from build123d import *

# Parameters (mm, degrees)
BOSS_EXTRUDE1_DEPTH      = 2
BOSS_EXTRUDE1_DEPTH_BACK = 5
SKETCH3_R                = 4
BOSS_EXTRUDE2_DEPTH      = 5
BOSS_EXTRUDE2_DEPTH_BACK = 2
SKETCH2_R                = 4
BOSS_EXTRUDE3_START      = -13.929206
SKETCH4_R                = 3.5
BOSS_EXTRUDE3_DEPTH      = 27.858412
CUT_EXTRUDE1_DEPTH       = 29.057975838
CUT_EXTRUDE1_DEPTH_BACK  = 5
SKETCH5_R                = 3
CUT_EXTRUDE2_DEPTH       = 29.057975747
CUT_EXTRUDE2_DEPTH_BACK  = 5
SKETCH6_R                = 3
SKETCH7_R                = 1.6
CUT_EXTRUDE3_DEPTH       = 33.668792587
SKETCH8_R                = 1.6
CUT_EXTRUDE4_DEPTH       = 33.668792494
SPLIT1_START             = -4.0000001
SPLIT1_OUTLINE_W         = 20
SPLIT1_OUTLINE_H         = 8.75
SPLIT1_DEPTH             = 0.5000001
SPLIT1_START_2           = 3.5
SPLIT1_2_OUTLINE_W       = 20
SPLIT1_2_OUTLINE_H       = 8.75
SPLIT1_2_DEPTH           = 0.5
SPLIT1_START_3           = -16.25
SPLIT1_3_DEPTH           = 7
SPLIT1_START_4           = 9.25
SPLIT1_4_DEPTH           = 7
SPLIT1_5_DEPTH           = 7
SPLIT1_6_DEPTH           = 7


# Read off the part's stored shape, not the designer's step: Split1
with BuildPart() as part:
    # Sketch3 → Boss-Extrude1 (new, two sides: drawn at the far end of the back side and taken through both)
    with BuildSketch(Plane(origin=(-7, 0, 14.25), x_dir=(1, 0, 0), z_dir=(0, 0, 1)).offset(-BOSS_EXTRUDE1_DEPTH_BACK)):
        Circle(SKETCH3_R)
    extrude(amount=BOSS_EXTRUDE1_DEPTH + BOSS_EXTRUDE1_DEPTH_BACK)



with BuildPart() as body_2:
    # Sketch2 → Boss-Extrude2 (new, two sides: drawn at the far end of the back side and taken through both)
    with BuildSketch(Plane(origin=(7, 0, -14.25), x_dir=(1, 0, 0), z_dir=(0, 0, 1)).offset(-BOSS_EXTRUDE2_DEPTH_BACK)):
        Circle(SKETCH2_R)
    extrude(amount=BOSS_EXTRUDE2_DEPTH + BOSS_EXTRUDE2_DEPTH_BACK)


with BuildPart() as part_1:
    add(part.part)

    add(body_2.part)  # Boss-Extrude3 merges body 2
    # Sketch4 → Boss-Extrude3 (add)
    with BuildSketch(Plane(origin=(0, 0, 0), x_dir=(-0.8975543264374148, 0, -0.44090387965346695), z_dir=(0.44090387965346695, 0, -0.8975543264374148)).offset(BOSS_EXTRUDE3_START)):
        with Locations(Location((0, 0, 0), (0, 0, 276.975190017))):
            Circle(SKETCH4_R)
    extrude(amount=BOSS_EXTRUDE3_DEPTH)

    # Sketch5 → Cut-Extrude1 (cut, two sides: drawn at the far end of the back side and taken through both)
    with BuildSketch(Plane.XY.offset(-9.25).offset(-CUT_EXTRUDE1_DEPTH_BACK)):
        with Locations(Location((7, 0, 0), (0, 0, 97.643118007))):
            Circle(SKETCH5_R)
    extrude(amount=CUT_EXTRUDE1_DEPTH + CUT_EXTRUDE1_DEPTH_BACK, mode=Mode.SUBTRACT)

    # Sketch6 → Cut-Extrude2 (cut, two sides: drawn at the far end of the back side and taken through both)
    with BuildSketch(Plane(origin=(0, 0, 9.25), x_dir=(-1, 0, 0), z_dir=(0, 0, -1)).offset(-CUT_EXTRUDE2_DEPTH_BACK)):
        with Locations(Location((7, 0, 0), (0, 0, 97.643118007))):
            Circle(SKETCH6_R)
    extrude(amount=CUT_EXTRUDE2_DEPTH + CUT_EXTRUDE2_DEPTH_BACK, mode=Mode.SUBTRACT)

    # Sketch7 → Cut-Extrude3 (cut, through all)
    with BuildSketch(Plane.XY.offset(-14.25)):
        with Locations((7, 0)):
            Circle(SKETCH7_R)
    extrude(amount=-CUT_EXTRUDE3_DEPTH, mode=Mode.SUBTRACT)

    # Sketch8 → Cut-Extrude4 (cut, through all)
    with BuildSketch(Plane(origin=(0, 0, 14.25), x_dir=(-1, 0, 0), z_dir=(0, 0, -1))):
        with Locations((7, 0)):
            Circle(SKETCH8_R)
    extrude(amount=-CUT_EXTRUDE4_DEPTH, mode=Mode.SUBTRACT)

    # Split1 outline → Split1 (cut)
    with BuildSketch(Plane(origin=(0, 0, 0), x_dir=(1, 0, 0), z_dir=(0, 1, 0)).offset(SPLIT1_START)):
        with Locations((0, -13.625)):
            Rectangle(SPLIT1_OUTLINE_W, SPLIT1_OUTLINE_H)
        with Locations((0, 13.625)):
            Rectangle(SPLIT1_OUTLINE_W, SPLIT1_OUTLINE_H)
    extrude(amount=SPLIT1_DEPTH, mode=Mode.SUBTRACT)

    # Split1 2 outline → Split1 2 (cut)
    with BuildSketch(Plane(origin=(0, 0, 0), x_dir=(1, 0, 0), z_dir=(0, 1, 0)).offset(SPLIT1_START_2)):
        with Locations((0, -13.625)):
            Rectangle(SPLIT1_2_OUTLINE_W, SPLIT1_2_OUTLINE_H)
        with Locations((0, 13.625)):
            Rectangle(SPLIT1_2_OUTLINE_W, SPLIT1_2_OUTLINE_H)
    extrude(amount=SPLIT1_2_DEPTH, mode=Mode.SUBTRACT)


with BuildPart() as body_2_2:
    # Split1 3 outline → Split1 3 (new body)
    with BuildSketch(Plane.XY.offset(SPLIT1_START_3)):
        with BuildLine():
            ThreePointArc((5.063508327, -3.5), (7, -4), (8.936491673, -3.5))
            Line((8.936491673, -3.5), (5.063508327, -3.5))
        make_face()
    extrude(amount=SPLIT1_3_DEPTH)


with BuildPart() as body_3:
    # Split1 4 outline → Split1 4 (new body)
    with BuildSketch(Plane.XY.offset(SPLIT1_START_4)):
        with BuildLine():
            ThreePointArc((-8.936491673, -3.5), (-7, -4), (-5.063508327, -3.5))
            Line((-5.063508327, -3.5), (-8.936491673, -3.5))
        make_face()
    extrude(amount=SPLIT1_4_DEPTH)


with BuildPart() as body_4:
    # Split1 5 outline → Split1 5 (new body)
    with BuildSketch(Plane.XY.offset(SPLIT1_START_4)):
        with BuildLine():
            Line((-8.936491673, 3.5), (-5.063508327, 3.5))
            ThreePointArc((-5.063508327, 3.5), (-7, 4), (-8.936491673, 3.5))
        make_face()
    extrude(amount=SPLIT1_5_DEPTH)


with BuildPart() as body_5:
    # Split1 6 outline → Split1 6 (new body)
    with BuildSketch(Plane.XY.offset(SPLIT1_START_3)):
        with BuildLine():
            Line((5.063508327, 3.5), (8.936491673, 3.5))
            ThreePointArc((8.936491673, 3.5), (7, 4), (5.063508327, 3.5))
        make_face()
    extrude(amount=SPLIT1_6_DEPTH)


solid = part_1.part
Can you work these out from the model? Positions are in its coordinate system, mm. A direction names the side the tool comes from. Round coordinates to 2 decimals unless told otherwise and drop trailing zeros. Loops run counter-clockwise (first coordinate to the right, second up) from the corner with the lowest first, then second, coordinate; pieces in that order, holes last. Notation, with made-up numbers: (39, 30) - (78, 30) arc R8 cw to (78, 35) - close; hole circle Ø1 at (-3, -4). An arc over 180 degrees is marked (long way). Answer in a Markdown table with one row per item. Add a question column.
Q1. We'd pull the mould along X, two halves only. Please class faces 6 (the cylindrical face through (-1.386, -3.186, -0.464)), 7 (the flat face through (7, -3.5, -13)), 8 (the flat face through (8.1, 1.5, -14.25)): pulls with the +X half, pulls with the -X half, needs draft (parallel to the pull), parting line crosses it, or undercut.
Q2. I want a section at B-B on y = 0. List the corners of the cut face in (x, z) for me, and give its area (3 significant figures).
Q3. I want a section at A-A on x = -7. List the corners of the cut face in (y, z) for me.
Q4. I want a section at D-D on y = 2.5. List the corners of the cut face in (x, z) for me.
Q5. For pin 1 Ø1.8 at (x, y) = (6, -0.5) entering from +Z; pin 2 Ø2.5 at (x, y) = (7, 0) entering from -Z; pin 3 Ø2 at (y, z) = (2, 10) entering from -X, each with a flat end and sliding along its axis, tell me the tip position at first contact or that it passes through.
Q6. I need wall thicknesses on L1, parallel to Y at x = 7, z = -15.65; L2, parallel to Z at x = -8, y = -2; L3, parallel to Z at x = 9, y = -1. Which ranges of each line are inside material? Lowest first, please.
Q7. I want a section at C-C on x = 7.5. List the corners of the cut face in (y, z) for me, and give its area (3 significant figures).
Q8. Which directions (+Z, -Z, +X, -X, +Y, -Y) give clear straight access to the entire face, cutting with the end or side of a thin tool? Please do faces 1 (the cylindrical face through (4.104, -0.783, -10.442)), 2 (the cylindrical face through (3, 0, -15)), 3 (the cylindrical face through (-3, 0, 15)), 4 (the cylindrical face through (-4.104, -0.783, 10.442)), 5 (the flat face through (7, 2, -16.25)).
A:
| question | item | result |
|---|---|---|
| 1 | face 6 | parting line crosses it |
| 1 | face 7 | needs draft |
| 1 | face 8 | undercut |
| 2 | outline | (-11, 9.25) - (-10, 9.25) - (-10, 14.25) - (-8.6, 14.25) - (-8.6, 16.25) - (-11, 16.25) - close; (-5.4, 14.25) - (-4, 14.25) - (-4, 0.2) - (3, -14.05) - (3, -16.25) - (5.4, -16.25) - (5.4, -14.25) - (4, -14.25) - (4, -0.2) - (-3, 14.05) - (-3, 16.25) - (-5.4, 16.25) - close; (8.6, -16.25) - (11, -16.25) - (11, -9.25) - (10, -9.25) - (10, -14.25) - (8.6, -14.25) - close |
| 2 | area | 155 mm^2 |
| 3 | outline | (-3.5, 9.25) - (-3, 9.25) - (-3, 14.25) - (-1.6, 14.25) - (-1.6, 16.25) - (-3.5, 16.25) - close; (1.6, 14.25) - (3, 14.25) - (3, 9.25) - (3.5, 9.25) - (3.5, 16.25) - (1.6, 16.25) - close |
| 4 | outline | (-10.12, 9.25) - (-8.66, 9.25) - (-8.66, 14.25) - (-5.34, 14.25) - (-5.34, 5.32) - (3.88, -13.45) - (3.88, -16.25) - (10.12, -16.25) - (10.12, -9.25) - (8.66, -9.25) - (8.66, -14.25) - (5.34, -14.25) - (5.34, -5.32) - (-3.88, 13.45) - (-3.88, 16.25) - (-10.12, 16.25) - close |
| 5 | pin 1 | z = -14.25 |
| 5 | pin 2 | through |
| 5 | pin 3 | x = -10.87 |
| 6 | L1 | -3.5 to -1.6, 1.6 to 3.5 |
| 6 | L2 | 14.25 to 16.25 |
| 6 | L3 | -16.25 to -14.25 |
| 7 | outline | (-3.5, -16.25) - (-1.52, -16.25) - (-1.52, -14.25) - (-2.96, -14.25) - (-2.96, -9.25) - (-3.5, -9.25) - close; (1.52, -16.25) - (3.5, -16.25) - (3.5, -9.25) - (2.96, -9.25) - (2.96, -14.25) - (1.52, -14.25) - close |
| 7 | area | 13.3 mm^2 |
| 8 | face 1 | +Z |
| 8 | face 2 | -Z, -X |
| 8 | face 3 | +Z, +X |
| 8 | face 4 | -Z |
| 8 | face 5 | -Z, +X, -X, +Y, -Y |
